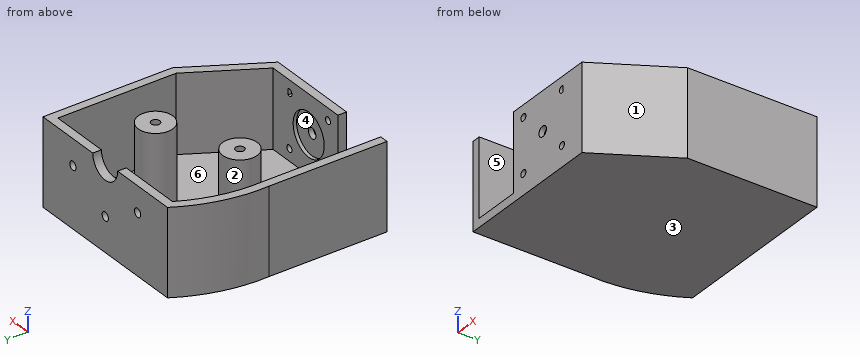
Autodesk Inventor part; units mm, degrees
ref_plane "YZ Plane" through (0, 0, 0) normal (1, 0, 0) x (0, 1, 0)
ref_plane "XZ Plane" through (0, 0, 0) normal (0, 1, 0) x (-1, 0, 0)
ref_plane "XY Plane" through (0, 0, 0) normal (0, 0, 1) x (1, 0, 0)
sketch "Sketch1" plane through (0, 0, 0) normal (0, 0, 1) x (1, 0, 0)
  line L0 (0, 0) -> (100, 0)
  line L1 (100, 0) -> (100, -75)
  line L2 (100, -75) -> (75, -118.3013)
  line L3 (-12.5, -50) -> (-12.5, -118.3013)
  arc A0 (0, 0) -> (-12.5, -50) centre (77.4072, -45.9143) ccw
  line L4 (-12.5, -118.3013) -> (75, -118.3013)
  dimension "d0" = 100
  dimension "d1" = 75
  dimension "d2" = 50
  dimension "d3" = 150
  dimension "d4" = 12.5
  dimension "d5" = 50
  dimension "d6" = 90
extrude "Extrusion1" add sketch "Sketch1" along normal blind 50
sketch "Sketch2" plane through (0, 0, 50) normal (0, 0, 1) x (1, 0, 0)
  line L0 (100, 0) -> (0, 0)
  arc A0 (0, 0) -> (-12.5, -50) centre (77.4072, -45.9143) ccw
  line L1 (-12.5, -50) -> (-12.5, -118.3013)
  line L2 (-12.5, -118.3013) -> (75, -118.3013)
  line L3 (75, -118.3013) -> (100, -75)
  line L4 (100, -75) -> (100, 0)
  arc A1 (2.902, -5) -> (-7.5, -49.8848) centre (77.4072, -45.9143) ccw
  line L5 (2.902, -5) -> (95, -5)
  line L6 (95, -5) -> (95, -73.6603)
  line L7 (95, -73.6603) -> (72.1132, -113.3013)
  line L8 (72.1132, -113.3013) -> (-7.5, -113.3013)
  line L9 (-7.5, -113.3013) -> (-7.5, -49.8848)
  dimension "d9" = 5
extrude "Extrusion2" cut sketch "Sketch2" against normal blind 45 contours L5 L6 L7 L8 L9 A1
sketch "Sketch3" plane through (0, 0, 50) normal (0, 0, 1) x (1, 0, 0)
  line L0 (72.1132, -113.3013) -> (-7.5, -113.3013)
  line L1 (-12.5, -118.3013) -> (75, -118.3013)
  line L2 (-7.5, -113.3013) -> (60, -113.3013)
  line L3 (60, -113.3013) -> (60, -118.3013)
  line L4 (60, -118.3013) -> (-7.5, -118.3013)
  line L5 (-7.5, -118.3013) -> (-7.5, -113.3013)
  point P0 (0, 0)
  dimension "d13" = 15
extrude "Extrusion3" cut sketch "Sketch3" against normal blind 45
sketch "Sketch4" plane through (0, 0, 0) normal (0, 1, 0) x (1, 0, 0)
  circle A0 centre (50, -50) radius 10
  line L0 (100, -50) -> (0, -50)
  point P0 (0, 0)
  dimension "d16" = 20
extrude "Extrusion4" cut sketch "Sketch4" against normal through all
sketch "Sketch5" plane through (0, 0, 0) normal (0, 1, 0) x (1, 0, 0)
  arc A0 (60, -50) -> (40, -50) centre (50, -50) ccw
  circle A1 centre (50, -50) radius 30 construction
  circle A2 centre (50, -20) radius 2.5
  circle A3 centre (24.0192, -35) radius 2.5
  circle A4 centre (24.0192, -65) radius 2.5
  circle A5 centre (50, -80) radius 2.5
  circle A6 centre (75.9808, -65) radius 2.5
  circle A7 centre (75.9808, -35) radius 2.5
  point P0 (0, 0)
  dimension "d20" = 60
  dimension "d21" = 5
  dimension "d24" = 360
extrude "Extrusion5" cut sketch "Sketch5" against normal blind 5 contours A2 | A3 | A7
sketch "Sketch17" plane through (-12.5, -118.3013, 0) normal (0, -1, 0) x (1, 0, 0)
  line L0 (72.5, 5) -> (32.5, 5)
  line L1 (32.5, 5) -> (32.5, 15)
  line L2 (32.5, 15) -> (72.5, 15)
  line L3 (72.5, 15) -> (72.5, 5)
  point P0 (12.5, 0)
  dimension "d68" = 40
  dimension "d69" = 10
extrude "Extrusion16" add sketch "Sketch17" against normal blind 5
sketch "Sketch18" plane through (0, 0, 5) normal (0, 0, 1) x (1, 0, 0)
  circle A0 centre (65, -40) radius 10
  circle A1 centre (65, -40) radius 2.5
  line L0 (100, 0) -> (0, 0)
  line L1 (100, -75) -> (100, 0)
  circle A2 centre (22.5, -58.3013) radius 10
  circle A3 centre (22.5, -58.3013) radius 2.5
  line L2 (-12.5, -50) -> (-12.5, -118.3013)
  line L3 (20, -118.3013) -> (60, -118.3013)
  point P0 (57.5, 0)
  dimension "d72" = 20
  dimension "d73" = 5
  dimension "d74" = 40
  dimension "d75" = 35
  dimension "d76" = 20
  dimension "d77" = 5
  dimension "d78" = 35
  dimension "d79" = 60
extrude "Extrusion17" add sketch "Sketch18" along normal blind 45
sketch "Sketch19" plane through (72.1132, -113.3013, 50) normal (0, 1, 0) x (1, 0, 0)
  line L0 (-52.1132, 45) -> (-5.1132, 45)
  line L1 (-5.1132, 45) -> (-5.1132, 0)
  line L2 (-5.1132, 0) -> (-52.1132, 0)
  line L3 (-52.1132, 0) -> (-52.1132, 45)
  line L4 (-13.1132, 38) -> (-44.1132, 38) construction
  line L5 (-44.1132, 38) -> (-44.1132, 7) construction
  line L6 (-44.1132, 7) -> (-13.1132, 7) construction
  line L7 (-13.1132, 7) -> (-13.1132, 38) construction
  circle A0 centre (-13.1132, 38) radius 2
  circle A1 centre (-13.1132, 7) radius 2
  circle A2 centre (-44.1132, 7) radius 2
  circle A3 centre (-44.1132, 38) radius 2
  circle A4 centre (-28.6132, 22.5) radius 3
  line L8 (-12.1132, 0) -> (-12.1132, 35)
  point P0 (-72.1132, 50)
  point P1 (-28.6132, 7)
  point P2 (-28.6132, 0)
  point P3 (-5.1132, 22.5)
  point P4 (-13.1132, 22.5)
  dimension "d82" = 31
  dimension "d83" = 31
  dimension "d84" = 4
  dimension "d85" = 4
  dimension "d86" = 4
  dimension "d87" = 4
  dimension "d88" = 6
  dimension "d96" = 7
extrude "Extrusion18" add sketch "Sketch19" against normal blind 5
extrude "Extrusion19" cut sketch "Sketch19" against normal blind 5 contours A0 | A3
sketch "Sketch20" plane through (72.1132, -113.3013, 50) normal (0, 1, 0) x (1, 0, 0)
  circle A0 centre (-28.6132, 22.5) radius 3
  circle A1 centre (-28.6132, 22.5) radius 12.5
  point P0 (-72.1132, 50)
  dimension "d93" = 25
extrude "Extrusion20" cut sketch "Sketch20" against normal blind 2
properties part number "FA001" material "ABS Plastic"
Model file for the job. Use its own axes, mm. Face numbers are marked on the shaded views. A direction names the side the tool comes from. Give positions to 0.01 mm unless a question says otherwise; leave off trailing zeros. Write each loop counter-clockwise with the first axis right and the second up, starting at its lowest first coordinate (ties: lowest second). Pieces come first, ordered by that corner, then holes. Notation, with made-up numbers: M 64,-36 L 68,-36 A35 cw 68,3 Z; hole C 25,33.25 d8. An arc over 180 degrees is marked long. One line per item, written item: value. Start each with the question number.
Q1. Saw through at C-C, the plane x = 65. Write the cut outline in (y, z), plus the area to 3 significant figures.
Q2. Saw through at A-A, the plane z = 35. State how many separate pieces and enclosed holes the cut face has, plus the area to 3 significant figures.
Q3. Saw through at D-D, the plane y = -87.5. Write the cut outline in (x, z), plus the area to 3 significant figures.
Q4. 3-axis set-ups, long thin cutter, end or side, ignore diameter. For the marked faces 4, 5 and 6: which of +Z, -Z, +X, -X, +Y, -Y reach the whole face in a straight line?
Q5. Two-plate mould, pull along X, no slides. Class the marked faces 1, 2 and 3: +X half, -X half, draft (parallel to the pull), parting line (faces both ways), or undercut.
Q6. Drop flat-ended pins along their axis: pin 1 Ø2.5 at (x, z) = (59, 12) entering from -Y; pin 2 Ø2.5 at (x, z) = (28, 43) entering from -Y; pin 3 Ø2 at (y, z) = (-101.5, 7.5) entering from -X. Give the stop position or say it passes through.
Q7. Probe probe 1 along Z at (x, y) = (59, -116); probe 2 along Y at (x, z) = (34, 24.5); probe 3 along Y at (x, z) = (65.5, 8). List the from-to ranges inside material, lowest first. Write a range as [from, to].
Output values:
1. outline: M -118.3,0 L 0,0 L 0,50 L -5,50 L -5,5 L -30,5 L -30,50 L -37.5,50 L -37.5,5 L -42.5,5 L -42.5,50 L -50,50 L -50,5 L -113.3,5 L -113.3,50 L -118.3,50 Z
1. area: 1,720 mm²
2. separate pieces: 5
2. enclosed holes: 2
2. area: 2,430 mm²
3. outline: M -12.5,0 L 92.78,0 L 92.78,50 L 87.01,50 L 87.01,5 L -7.5,5 L -7.5,50 L -12.5,50 Z
3. area: 1,010 mm²
4. face 4: none
4. face 5: +Z, -Y
4. face 6: +Z
5. face 1: +X half
5. face 2: undercut
5. face 3: draft
6. pin 1: stops at y = -48.8
6. pin 2: stops at y = -67.35
6. pin 3: stops at x = -12.5
7. probe 1: z = [0, 10], [14, 41], [45, 50]
7. probe 2: y = [-118.3, -115.3], [-5, 0]
7. probe 3: y = [-118.3, -113.3], [-49.99, -42.45], [-37.55, -30.01], [-5, 0]
